Part print with two shaded views. Sizes in mm from the minimum x, y, z corner. A direction names the side the tool comes from. Round coordinates to 2 decimals unless told otherwise and drop trailing zeros. Order: outer loops, then holes, each group sorted by start corner. A loop starts at its lowest first (then second) coordinate and runs counter-clockwise, first axis right, second up. Notation, with made-up numbers: (37.25, 12) -> (45.25, 12) arc R9 ccw to (45.25, 23) -> close; hole circle Ø2 at (-28.75, 40). An arc over 180 degrees is marked (long way). Use a Markdown table: item, result. Add a question column.
Item 1: Two-plate mould, pull along Y, no slides. Class the marked faces 3, 4 and 5: released by +Y, released by -Y, zero draft, split by the parting line, or undercut.
Item 2: 3-axis set-ups, long thin cutter, end or side, ignore diameter. For the marked faces 1 and 2: which of +Z, -Z, +X, -X, +Y, -Y reach the whole face in a straight line?
Item 3: Slice it at B-B, the plane x = 19.9. Give the cut face in (y, z), plus the area to 3 significant figures.
Item 4: Slice it at D-D, the plane y = 5.5. Give the cut face in (x, z), plus the area to 3 significant figures.
Item 5: Probe L1, parallel to Y at x = 19.9, z = 0.75; L2, parallel to X at y = 2.25, z = 0.3; L3, parallel to Z at x = 11.25, y = 4. List the from-to ranges inside material, lowest first.
Item 6: Slice it at A-A, the plane z = 1.05. Give the cut face in (x, y).
Item 7: Slice it at C-C, the plane y = 3.9. Give the cut face in (x, z), plus the area to 3 significant figures.
Item 8: Pin check, flat tips, straight feed: pin 1 (4 mm diameter, centred on x = 20.5, y = 4.5, fed in from -Z); pin 2 (2.5 mm diameter, centred on x = 13, y = 4, fed in from -Z). Stop position of each tip, or through.
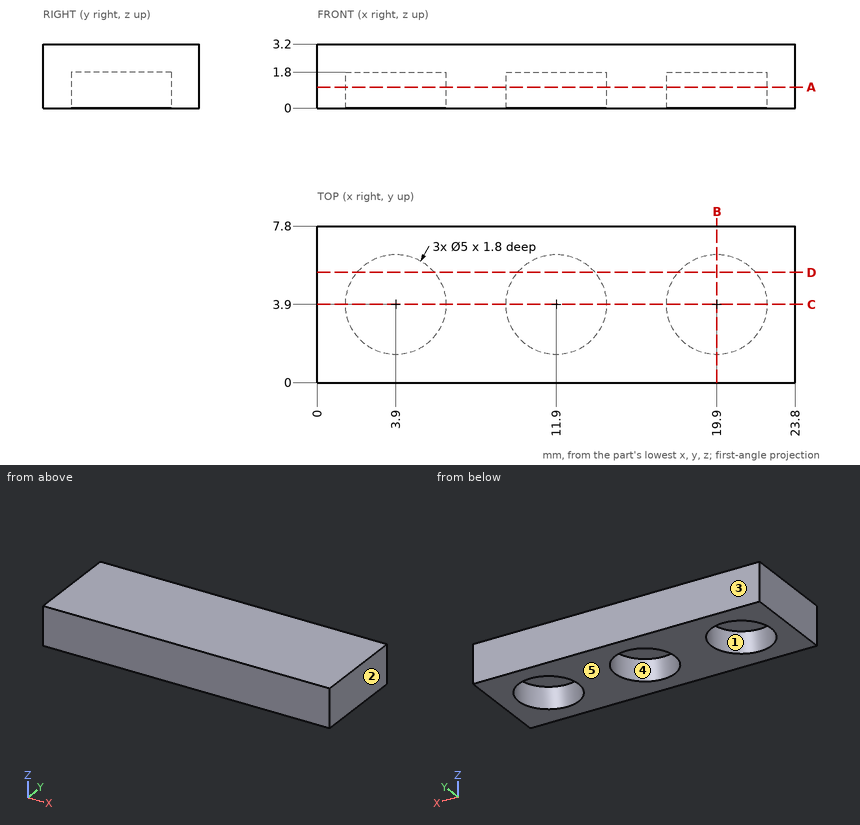
Check sheet entries:
| question | item | result |
|---|---|---|
| 1 | face 3 | released by +Y |
| 1 | face 4 | undercut |
| 1 | face 5 | zero draft |
| 2 | face 1 | -Z |
| 2 | face 2 | +Z, -Z, +X, +Y, -Y |
| 3 | outline | (0, 0) -> (1.4, 0) -> (1.4, 1.8) -> (6.4, 1.8) -> (6.4, 0) -> (7.8, 0) -> (7.8, 3.2) -> (0, 3.2) -> close |
| 3 | area | 16.0 mm2 |
| 4 | outline | (0, 0) -> (1.98, 0) -> (1.98, 1.8) -> (5.82, 1.8) -> (5.82, 0) -> (9.98, 0) -> (9.98, 1.8) -> (13.82, 1.8) -> (13.82, 0) -> (17.98, 0) -> (17.98, 1.8) -> (21.82, 1.8) -> (21.82, 0) -> (23.8, 0) -> (23.8, 3.2) -> (0, 3.2) -> close |
| 4 | area | 55.4 mm2 |
| 5 | L1 | 0 to 1.4, 6.4 to 7.8 |
| 5 | L2 | 0 to 2.02, 5.78 to 10.02, 13.78 to 18.02, 21.78 to 23.8 |
| 5 | L3 | 1.8 to 3.2 |
| 6 | outline | (0, 0) -> (23.8, 0) -> (23.8, 7.8) -> (0, 7.8) -> close; hole circle Ø5 at (3.9, 3.9); hole circle Ø5 at (11.9, 3.9); hole circle Ø5 at (19.9, 3.9) |
| 7 | outline | (0, 0) -> (1.4, 0) -> (1.4, 1.8) -> (6.4, 1.8) -> (6.4, 0) -> (9.4, 0) -> (9.4, 1.8) -> (14.4, 1.8) -> (14.4, 0) -> (17.4, 0) -> (17.4, 1.8) -> (22.4, 1.8) -> (22.4, 0) -> (23.8, 0) -> (23.8, 3.2) -> (0, 3.2) -> close |
| 7 | area | 49.2 mm2 |
| 8 | pin 1 | z = 0 |
| 8 | pin 2 | z = 1.8 |
